from build123d import *

# Parameters (mm, degrees)
SKETCH1_R           = 1.524
BOSS_EXTRUDE1_DEPTH = 1.5875
CHAMFER1_SIZE       = 1.7145
CHAMFER1_SIZE2      = 1.490392112


with BuildPart() as part:
    # Sketch1 → Boss-Extrude1 (new body)
    with BuildSketch(Plane(origin=(0, 0, 0), x_dir=(1, 0, 0), z_dir=(0, 1, 0))):
        with BuildLine():
            Line((-26.3525, -38.1), (26.3525, -38.1))
            ThreePointArc((26.3525, -38.1), (28.59756403, -37.17006403), (29.5275, -34.925))
            Line((29.5275, -34.925), (29.5275, -27.795278791))
            ThreePointArc((29.5275, -27.795278791), (29.294536895, -26.732649616), (28.638381288, -25.864944371))
            Line((28.638381288, -25.864944371), (26.334171426, -23.89431332))
            ThreePointArc((26.334171426, -23.89431332), (25.678015818, -23.026608076), (25.445052714, -21.9639789))
            Line((25.445052714, -21.9639789), (25.445052714, 21.9639789))
            ThreePointArc((25.445052714, 21.9639789), (25.678015818, 23.026608076), (26.334171426, 23.89431332))
            Line((26.334171426, 23.89431332), (28.638381288, 25.864944371))
            ThreePointArc((28.638381288, 25.864944371), (29.294536895, 26.732649616), (29.5275, 27.795278791))
            Line((29.5275, 27.795278791), (29.5275, 30.48))
            ThreePointArc((29.5275, 30.48), (27.295653673, 35.868153673), (21.9075, 38.1))
            Line((21.9075, 38.1), (-21.9075, 38.1))
            ThreePointArc((-21.9075, 38.1), (-27.295653673, 35.868153673), (-29.5275, 30.48))
            Line((-29.5275, 30.48), (-29.5275, 27.795278791))
            ThreePointArc((-29.5275, 27.795278791), (-29.294536895, 26.732649616), (-28.638381288, 25.864944371))
            Line((-28.638381288, 25.864944371), (-26.334171426, 23.89431332))
            ThreePointArc((-26.334171426, 23.89431332), (-25.678015818, 23.026608076), (-25.445052714, 21.9639789))
            Line((-25.445052714, 21.9639789), (-25.445052714, -21.9639789))
            ThreePointArc((-25.445052714, -21.9639789), (-25.678015818, -23.026608076), (-26.334171426, -23.89431332))
            Line((-26.334171426, -23.89431332), (-28.638381288, -25.864944371))
            ThreePointArc((-28.638381288, -25.864944371), (-29.294536895, -26.732649616), (-29.5275, -27.795278791))
            Line((-29.5275, -27.795278791), (-29.5275, -34.925))
            ThreePointArc((-29.5275, -34.925), (-28.59756403, -37.17006403), (-26.3525, -38.1))
        make_face()
        with Locations((24.4475, 33.02)):
            Circle(SKETCH1_R, mode=Mode.SUBTRACT)
        with Locations((-24.4475, -33.02)):
            Circle(SKETCH1_R, mode=Mode.SUBTRACT)
        with Locations((-24.4475, 33.02)):
            Circle(SKETCH1_R, mode=Mode.SUBTRACT)
        with Locations((24.4475, -33.02)):
            Circle(SKETCH1_R, mode=Mode.SUBTRACT)
    extrude(amount=BOSS_EXTRUDE1_DEPTH)

    # Chamfer1
    chamfer1_edges = [part.edges().sort_by_distance(p)[0] for p in [
        (22.9235, 0, -33.02),
        (-25.9715, 0, 33.02),
        (-25.9715, 0, -33.02),
        (22.9235, 0, 33.02),
    ]]
    chamfer1_side = [part.faces().sort_by_distance(p)[0] for p in [
        (0, 0, 0.184699289),
    ]]
    chamfer(chamfer1_edges, length=CHAMFER1_SIZE, length2=CHAMFER1_SIZE2, reference=chamfer1_side[0])


solid = part.part
Input: part model. Units: mm. Frame: model coordinates. A direction names the side the tool comes from. Give positions to 0.01 mm unless a question says otherwise; leave off trailing zeros. Write each loop counter-clockwise with the first axis right and the second up, starting at its lowest first coordinate (ties: lowest second). Pieces come first, ordered by that corner, then holes. Notation, with made-up numbers: (42.25, 68) -> (75.25, 68) arc R22 ccw to (75.25, 79) -> close; hole circle Ø8 at (85.25, 69.25). An arc over 180 degrees is marked (long way). Use one line per item in the form item = value. Start each with the question number.
1) Section query B-B on y = 1.2. Count the separate pieces of the cut face and the enclosed holes in it, then the cut area to 3 significant figures.
2) Pin query (flat end, axial travel): pin 1 (2.5 mm diameter, centred on x = 24.45, z = -33.02, fed in from -Y); pin 2 (1.5 mm diameter, centred on x = -7.5, z = -5.5, fed in from -Y); pin 3 (4 mm diameter, centred on x = -24.45, z = -33.02, fed in from -Y); pin 4 (0.5 mm diameter, centred on y = 1, z = 8, fed in from -X). Return the tip coordinate at first contact, or that it passes through.
3) Section query D-D on z = 16.5. Return the cut outline in (x, y).
4) Section query C-C on z = -33.02. Return the cut outline in (x, y), then the cut area to 3 significant figures.
5) Section query A-A on z = 33.02. Return the cut outline in (x, y).
6) Set-up query: faces 5 (the flat face through (-25.445, 1, 0)), 6 (the cylindrical face through (25.684, 0.783, 23.041)), 7 (the cylindrical face through (-28.62, 0.78, 37.15)). Return all of +Z, -Z, +X, -X, +Y, -Y with unobstructed straight access to the full face (end or side cutting, diameter ignored); none if empty.
7) Draft query along Z for faces 1 (the flat face through (-29.528, 1, -29)), 2 (the cylindrical face through (-25.67, 0.78, 23.01)), 3 (the cylindrical face through (-27.236, 0.783, -35.927)), 4 (the flat face through (0, 1, 38.1)). Return one class per face: pulls with the +Z half, pulls with the -Z half, needs draft (parallel to the pull), parting line crosses it, or undercut.
8) Ray query, probe 1 along X at (y, z) = (1.55, 33.02); probe 2 along X at (y, z) = (1.2, -34.5); probe 3 along Z at (x, y) = (-24.5, 1.25). Return the intervals inside material, ascending. Write a range as from..to.
Outcome:
q1.separate_pieces = 1
q1.enclosed_holes = 4
q1.area = 4,020 mm^2
q2.pin_1 = through
q2.pin_2 = 0
q2.pin_3 = 1.07
q2.pin_4 = -25.45
q3.outline = (-25.45, 0) -> (25.45, 0) -> (25.45, 1.59) -> (-25.45, 1.59) -> close
q4.outline = (-29.09, 0) -> (-27.69, 0) -> (-25.97, 1.49) -> (-25.97, 1.59) -> (-29.09, 1.59) -> close; (-22.92, 1.49) -> (-21.21, 0) -> (21.21, 0) -> (22.92, 1.49) -> (22.92, 1.59) -> (-22.92, 1.59) -> close; (25.97, 1.49) -> (27.69, 0) -> (29.09, 0) -> (29.09, 1.59) -> (25.97, 1.59) -> close
q4.area = 77.6 mm^2
q5.outline = (-29.53, 0) -> (-27.69, 0) -> (-25.97, 1.49) -> (-25.97, 1.59) -> (-29.53, 1.59) -> close; (-22.92, 1.49) -> (-21.21, 0) -> (21.21, 0) -> (22.92, 1.49) -> (22.92, 1.59) -> (-22.92, 1.59) -> close; (25.97, 1.49) -> (27.69, 0) -> (29.53, 0) -> (29.53, 1.59) -> (25.97, 1.59) -> close
q6.face_5 = -X, +Y, -Y
q6.face_6 = +X, +Y, -Y
q6.face_7 = +Z, -X, +Y, -Y
q7.face_1 = needs draft
q7.face_2 = undercut
q7.face_3 = pulls with the -Z half
q7.face_4 = pulls with the +Z half
q8.probe_1 = -29.53..-25.97, -22.92..22.92, 25.97..29.53
q8.probe_2 = -28.38..-25.57, -23.32..23.32, 25.57..28.38
q8.probe_3 = -37.65..-34.82, -31.22..31.22, 34.82..38.1
